Work out the finished part from the listing and answer in its coordinate system (mm). Face numbers are marked on the shaded views. A direction names the side the tool comes from. Coordinates: 2 decimals unless noted, no trailing zeros. Order: outer loops, then holes, each group sorted by start corner. A loop starts at its lowest first (then second) coordinate and runs counter-clockwise, first axis right, second up.
1. Determine the mould class of the marked faces 3, 4 and 5 for opening direction X: +X half, -X half, draft (parallel to the pull), parting line (faces both ways), or undercut.
2. The part is cut by section C-C, the plane z = 7.75. Give the vertices of the cut face in (x, y).
3. Find the intervals of material crossed by probe 1 along X at (y, z) = (2.25, 6.25); probe 2 along X at (y, z) = (6.5, 7.5); probe 3 along Z at (x, y) = (10.75, 7.25), in increasing order.
4. The part is cut by section B-B, the plane y = 8.25. Give the vertices of the cut face in (x, z).
5. The part is cut by section D-D, the plane z = 5.25. Give the vertices of the cut face in (x, y), then the cut area to 3 significant figures.
6. Flat-ended cylindrical pins translate along their axes: pin 1 Ø3 at (x, z) = (15.5, 5.5) entering from +Y; pin 2 Ø3 at (x, y) = (9, 2) entering from +Z; pin 3 Ø3.5 at (x, y) = (6.5, 9) entering from +Z. Find the tip coordinate at first contact, or state that the pin passes through.
7. A tool of negligible diameter and unlimited length cuts with its end or side. For the marked faces 1 and 2, from which of +Z, -Z, +X, -X, +Y, -Y can it reach the whole face along a straight path? Write none if from no direction.
8. The part is cut by section A-A, the plane x = 19. Give the vertices of the cut face in (y, z).
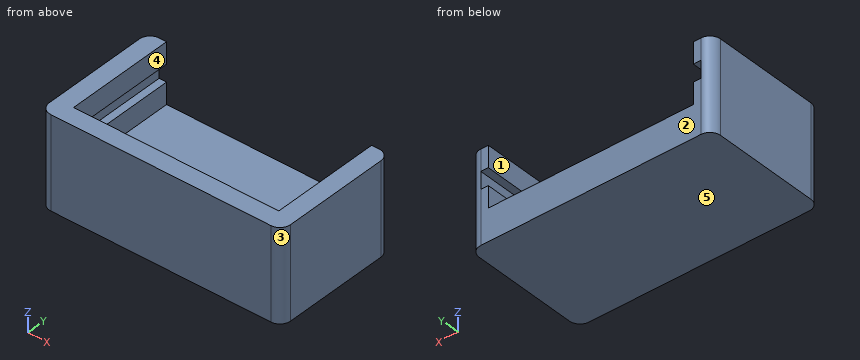
```python
from build123d import *

# Parameters (mm, degrees)
BOX007_W     = 20.6
BOX007_H     = 11
BOX007_DEPTH = 1.6
BOX006_W     = 19.2
BOX006_H     = 10.6
BOX006_DEPTH = 5.6
BOX_W        = 22.6
BOX_H        = 12
BOX_DEPTH    = 8.6
FILLET_R     = 1


with BuildPart() as pcb_extract_cube:
    # Box007 → Box007 (new body)
    with BuildSketch(Plane(origin=(1, 1, 5), x_dir=(1, 0, 0), z_dir=(0, 0, 1))):
        with Locations((10.3, 5.5)):
            Rectangle(BOX007_W, BOX007_H)
    extrude(amount=BOX007_DEPTH)


with BuildPart() as extract_fusion:
    # Box006 → Box006 (new body)
    with BuildSketch(Plane(origin=(1.7, 1.7, 3), x_dir=(1, 0, 0), z_dir=(0, 0, 1))):
        with Locations((9.6, 5.3)):
            Rectangle(BOX006_W, BOX006_H)
    extrude(amount=BOX006_DEPTH)

    # Fusion: union pcb extract cube
    add(pcb_extract_cube.part)


with BuildPart() as obj1:
    # Box → Box (new body)
    with BuildSketch(Plane.XY):
        with Locations((11.3, 6)):
            Rectangle(BOX_W, BOX_H)
    extrude(amount=BOX_DEPTH)

    # Fillet
    fillet_edges = [obj1.edges().sort_by_distance(p)[0] for p in [
        (0, 0, 4.3),
        (0, 12, 4.3),
        (22.6, 0, 4.3),
        (22.6, 12, 4.3),
    ]]
    fillet(fillet_edges, radius=FILLET_R)

    # Cut003006: cut extract fusion
    add(extract_fusion.part, mode=Mode.SUBTRACT)


solid = obj1.part
```
Geometry says:
1. face 3: +X half
1. face 4: undercut
1. face 5: draft
2. outline: (0, 1) arc R1 ccw to (1, 0) - (21.6, 0) arc R1 ccw to (22.6, 1) - (22.6, 11) arc R1 ccw to (21.6, 12) - (20.9, 12) - (20.9, 1.7) - (1.7, 1.7) - (1.7, 12) - (1, 12) arc R1 ccw to (0, 11) - close
3. probe 1: x = 0 to 1, 21.6 to 22.6
3. probe 2: x = 0 to 1.7, 20.9 to 22.6
3. probe 3: z = 0 to 3
4. outline: (0, 0) - (22.6, 0) - (22.6, 8.6) - (20.9, 8.6) - (20.9, 6.6) - (21.6, 6.6) - (21.6, 5) - (20.9, 5) - (20.9, 3) - (1.7, 3) - (1.7, 5) - (1, 5) - (1, 6.6) - (1.7, 6.6) - (1.7, 8.6) - (0, 8.6) - close
5. outline: (0, 1) arc R1 ccw to (1, 0) - (21.6, 0) arc R1 ccw to (22.6, 1) - (22.6, 11) arc R1 ccw to (21.6, 12) - (21.6, 1) - (1, 1) - (1, 12) arc R1 ccw to (0, 11) - close
5. area: 43.7 mm2
6. pin 1: stops at y = 1.7
6. pin 2: stops at z = 8.6
6. pin 3: stops at z = 3
7. face 1: +Z, +Y
7. face 2: +Z, -Z, +X, -X, +Y
8. outline: (0, 0) - (12, 0) - (12, 3) - (1.7, 3) - (1.7, 5) - (1, 5) - (1, 6.6) - (1.7, 6.6) - (1.7, 8.6) - (0, 8.6) - close
